Check sheet for the drawn part. Datum: minimum x, y, z corner. Units: mm. A direction names the side the tool comes from. Give positions to 0.01 mm unless a question says otherwise; leave off trailing zeros. Loops run counter-clockwise (first coordinate to the right, second up) from the corner with the lowest first, then second, coordinate; pieces in that order, holes last. Notation, with made-up numbers: (-39, -19.75) - (-25, -19.75) arc R23 cw to (-25, -6.75) - close; hole circle Ø6 at (20, 68.5). An arc over 180 degrees is marked (long way). One line per item, written item: value. Start each with the question number.
1. Sectioned sample at D-D (x = 100.5). Record the cut outline in (y, z), plus the area to 3 significant figures.
2. Access from +Z, -Z, +X, -X, +Y, -Y to the whole of each face (thin tool, end or side, straight path). Record for the marked faces 1 and 2.
3. Mould release check, pull along Z, two halves, no side actions. Record for the marked faces 3, 4 and 5: pulls with the +Z half, pulls with the -Z half, needs draft (parallel to the pull), parting line crosses it, or undercut.
4. Sectioned sample at C-C (z = 20). Record the cut outline in (x, y), plus the area to 3 significant figures.
5. Sectioned sample at B-B (x = 160). Record the cut outline in (y, z).
6. Sectioned sample at A-A (z = 90). Record the cut outline in (x, y).
7. Scan lines: L1, parallel to Z at x = 160, y = 1.4; L2, parallel to X at y = 10.25, z = 90. Record each from-to range of solid material in increasing order. Write a range as [from, to].
8. Gauge pin test, flat ends, axial feed: pin 1 (6.5 mm diameter, centred on x = 160, z = 160, fed in from +Y); pin 2 (1 mm diameter, centred on x = 158.5, z = 113, fed in from +Y); pin 3 (12 mm diameter, centred on y = 17.5, z = 105.5, fed in from -X). Record the tip position at first contact, or that the pin passes through.
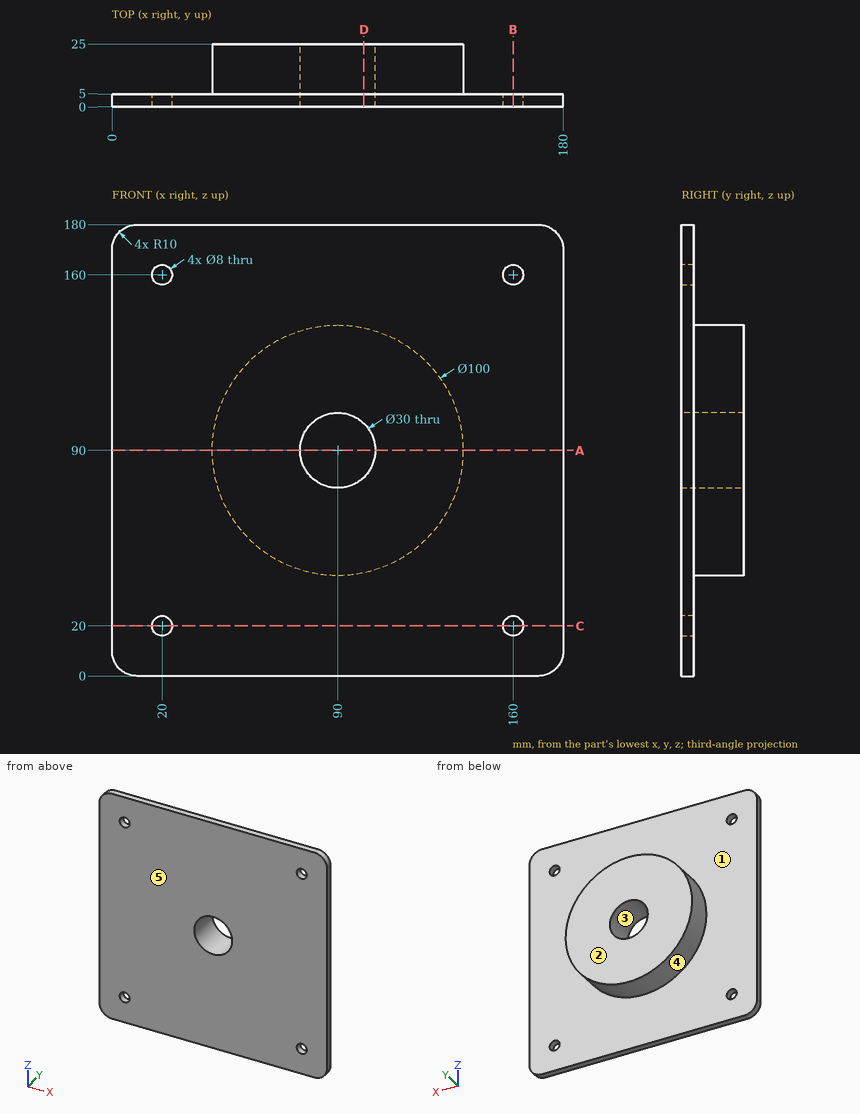
Results are:
1. outline: (0, 0) - (5, 0) - (5, 41.11) - (25, 41.11) - (25, 79.29) - (0, 79.29) - close; (0, 100.71) - (25, 100.71) - (25, 138.89) - (5, 138.89) - (5, 180) - (0, 180) - close
1. area: 2,320 mm^2
2. face 1: +Y
2. face 2: +Z, -Z, +X, -X, +Y
3. face 3: undercut
3. face 4: parting line crosses it
3. face 5: needs draft
4. outline: (0, 0) - (16, 0) - (16, 5) - (0, 5) - close; (24, 0) - (156, 0) - (156, 5) - (24, 5) - close; (164, 0) - (180, 0) - (180, 5) - (164, 5) - close
4. area: 820 mm^2
5. outline: (0, 0) - (5, 0) - (5, 16) - (0, 16) - close; (0, 24) - (5, 24) - (5, 156) - (0, 156) - close; (0, 164) - (5, 164) - (5, 180) - (0, 180) - close
6. outline: (0, 0) - (75, 0) - (75, 25) - (40, 25) - (40, 5) - (0, 5) - close; (105, 0) - (180, 0) - (180, 5) - (140, 5) - (140, 25) - (105, 25) - close
7. L1: z = [0, 16], [24, 156], [164, 180]
7. L2: x = [40, 75], [105, 140]
8. pin 1: passes through
8. pin 2: stops at y = 5
8. pin 3: stops at x = 40.91
